Geometry: final body of the model. Coordinates: model frame, mm. Face numbers are marked on the shaded views. A direction names the side the tool comes from. Coordinates: 2 decimals unless noted, no trailing zeros. Write each loop counter-clockwise with the first axis right and the second up, starting at its lowest first coordinate (ties: lowest second). Pieces come first, ordered by that corner, then holes. Notation, with made-up numbers: (3.5, 3) - (16.5, 3) arc R7 cw to (16.5, 10) - close; hole circle Ø7 at (-12, 34). An arc over 180 degrees is marked (long way). Answer as a JSON object with one key per item and string values. Group by question number.
Item 1: Set-up query: the marked faces 4, 5, 6, 7 and 8. Return all of +Z, -Z, +X, -X, +Y, -Y with unobstructed straight access to the full face (end or side cutting, diameter ignored); none if empty.
Item 2: Section B-B on y = 28.5. Return loops of the section in (x, z), and give its area (3 significant figures).
Item 3: Mould query, pull axis X, two halves, no side actions, for the marked faces 1, 2 and 3. Classes: pulls with the +X half, pulls with the -X half, needs draft (parallel to the pull), parting line crosses it, or undercut.
Item 4: Line query: line 1 along X through (y, z) = (44, 4); line 2 along X through (y, z) = (3, 5.25); line 3 along Y through (x, z) = (-27, 4.5). Output: solid intervals per line, ascending. Write a range as from..to.
Item 5: Section A-A on x = -22.5. Return loops of the section in (y, z).
Item 6: First-contact query: pin 1 Ø2 at (x, z) = (-20, 2) entering from +Y; pin 2 Ø3 at (x, z) = (-39.5, 3.5) entering from -Y; pin 3 Ø3 at (y, z) = (3, 3.5) entering from +X; pin 4 Ø3 at (y, z) = (3.5, 3) entering from -X. Flat tips, straight axial feed; report the tip coordinate or a pass-through.
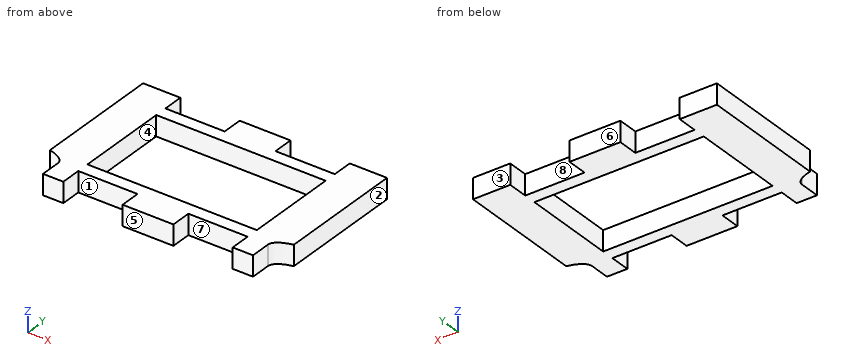
```python
from build123d import *

# Parameters (mm, degrees)
BOSS_EXTRUDE1_DEPTH = 6
SKETCH4_W           = 50
SKETCH4_H           = 27.629262186
CUT_EXTRUDE1_DEPTH  = 90.560035874


with BuildPart() as part:
    # Sketch2 → Boss-Extrude1 (new body)
    with BuildSketch(Plane.XY):
        with BuildLine():
            Line((-15, 0), (-9, 0))
            Line((-9, 0), (-9, 6))
            add(Edge.make_bspline(
                [(-4, 9.583225666), (-9, 8.480694692), (-9, 6)],
                knots=[5.172942972, 5.172942972, 5.172942972, 6.283185307, 6.283185307, 6.283185307], degree=2, weights=[1, 0.849836586, 1]))
            Line((-4, 9.583225666), (-4, 41))
            Line((-4, 41), (-4, 47))
            Line((-4, 47), (-15, 47))
            Line((-15, 47), (-15, 41))
            Line((-15, 41), (-32.5, 41))
            Line((-32.5, 41), (-32.5, 47))
            Line((-32.5, 47), (-47.5, 47))
            Line((-47.5, 47), (-47.5, 41))
            Line((-47.5, 41), (-65, 41))
            Line((-65, 41), (-65, 47))
            Line((-65, 47), (-76, 47))
            Line((-76, 47), (-76, 41))
            Line((-76, 41), (-76, 9.583225666))
            add(Edge.make_bspline(
                [(-71, 6), (-71, 8.480694692), (-76, 9.583225666)],
                knots=[0, 0, 0, 1.110242335, 1.110242335, 1.110242335], degree=2, weights=[1, 0.849836586, 1]))
            Line((-71, 6), (-71, 0))
            Line((-71, 0), (-65, 0))
            Line((-65, 0), (-65, 6))
            Line((-65, 6), (-47.5, 6))
            Line((-47.5, 6), (-47.5, 0))
            Line((-47.5, 0), (-32.5, 0))
            Line((-32.5, 0), (-32.5, 6))
            Line((-32.5, 6), (-15, 6))
            Line((-15, 6), (-15, 0))
        make_face()
    extrude(amount=BOSS_EXTRUDE1_DEPTH)

    # Sketch4 → Cut-Extrude1 (cut, through all)
    with BuildSketch(Plane(origin=(0, 0, 0), x_dir=(-1, 0, 0), z_dir=(0, 0, -1))):
        with Locations((40, 23.5)):
            Rectangle(SKETCH4_W, SKETCH4_H)
    extrude(amount=-CUT_EXTRUDE1_DEPTH, mode=Mode.SUBTRACT)


solid = part.part
```
Checks:
{
 "1": {"face 4": "+Z, -Z", "face 5": "+Z, -Z, +X, -X, -Y", "face 6": "+Z, -Z, +X, -X, +Y", "face 7": "+Z, -Z, -Y", "face 8": "+Z, -Z, +Y"},
 "2": {"outline": "(-76, 0) - (-65, 0) - (-65, 6) - (-76, 6) - close; (-15, 0) - (-4, 0) - (-4, 6) - (-15, 6) - close", "area": "132 mm^2"},
 "3": {"face 1": "undercut", "face 2": "pulls with the +X half", "face 3": "needs draft"},
 "4": {"line 1": "-76..-65, -47.5..-32.5, -15..-4", "line 2": "-71..-65, -47.5..-32.5, -15..-9", "line 3": "6..9.69, 37.31..41"},
 "5": {"outline": "(6, 0) - (9.69, 0) - (9.69, 6) - (6, 6) - close; (37.31, 0) - (41, 0) - (41, 6) - (37.31, 6) - close"},
 "6": {"pin 1": "y = 41", "pin 2": "y = 0", "pin 3": "x = -9", "pin 4": "x = -71"}
}
